The listing builds one solid part. Answer for the finished solid, in the listing's coordinates (mm). Give positions to 0.01 mm unless a question says otherwise; leave off trailing zeros. Write each loop counter-clockwise with the first axis right and the second up, starting at its lowest first coordinate (ties: lowest second). Pieces come first, ordered by that corner, then holes. Notation, with made-up numbers: (-29.75, 87.25) -> (20.25, 87.25) arc R16 cw to (20.25, 104.25) -> close; hole circle Ø3 at (68.5, 66). An arc over 180 degrees is marked (long way). One line per question, with ' | ' between items.
from build123d import *

# Parameters (mm, degrees)
BOSS_EXTRU_1_DEPTH = 1


with BuildPart() as part:
    # Esquisse1 → Boss.-Extru.1 (new body)
    with BuildSketch(Plane.XY):
        with BuildLine():
            Line((0, 0), (49, 0))
            Line((49, 0), (49, 22))
            ThreePointArc((49, 22), (41.824116139, 39.324116139), (24.5, 46.5))
            ThreePointArc((24.5, 46.5), (7.175883861, 39.324116139), (0, 22))
            Line((0, 22), (0, 0))
        make_face()
    extrude(amount=BOSS_EXTRU_1_DEPTH)


solid = part.part
Item 1: Consider line 1 (Y direction, x = 15, z = 0.1); line 2 (X direction, y = 42.5, z = 0.35); line 3 (Y direction, x = 31, z = 0.8). Determine where each line is inside the solid, lowest interval first. Write a range as [from, to].
Answers below:
line 1: [0, 44.58] | line 2: [11.08, 37.92] | line 3: [0, 45.62]
Item 2: Find section A-A (z = 0.2). Write down the section's boundary in (x, y), then the cut area to 3 significant figures.
Answers below:
outline: (0, 0) -> (49, 0) -> (49, 22) arc R24.5 ccw to (0, 22) -> close | area: 2,020 mm²
Item 3: Find section B-B (x = 8.5). Write down the section's boundary in (y, z).
Answers below:
outline: (0, 0) -> (40.55, 0) -> (40.55, 1) -> (0, 1) -> close
Item 4: Find section C-C (y = 39.5). Write down the section's boundary in (x, z), then the cut area to 3 significant figures.
Answers below:
outline: (7.35, 0) -> (41.65, 0) -> (41.65, 1) -> (7.35, 1) -> close | area: 34.3 mm²
